from build123d import *

# Parameters (mm, degrees)
SKETCH1_R           = 10
SKETCH1_R_2         = 1
SKETCH1_R_3         = 1.5
BOSS_EXTRUDE1_DEPTH = 2
SKETCH2_R           = 4.5
SKETCH2_R_2         = 3.025
BOSS_EXTRUDE2_DEPTH = 2.5


with BuildPart() as part:
    # Sketch1 → Boss-Extrude1 (new body)
    with BuildSketch(Plane.XY):
        Circle(SKETCH1_R)
        with Locations((7, 0)):
            Circle(SKETCH1_R_2, mode=Mode.SUBTRACT)
        with Locations((0, 7)):
            Circle(SKETCH1_R_2, mode=Mode.SUBTRACT)
        Circle(SKETCH1_R_3, mode=Mode.SUBTRACT)
        with Locations((0, -7)):
            Circle(SKETCH1_R_2, mode=Mode.SUBTRACT)
        with Locations((-7, 0)):
            Circle(SKETCH1_R_2, mode=Mode.SUBTRACT)
    extrude(amount=BOSS_EXTRUDE1_DEPTH)

    # Sketch2 → Boss-Extrude2 (add)
    with BuildSketch(Plane.XY.offset(2)):
        Circle(SKETCH2_R)
        Circle(SKETCH2_R_2, mode=Mode.SUBTRACT)
    extrude(amount=BOSS_EXTRUDE2_DEPTH)


solid = part.part
CAD build for the part. Positions are in the model's coordinates, mm. A direction names the side the tool comes from. Give positions to 0.01 mm unless a question says otherwise; leave off trailing zeros. Write each loop counter-clockwise with the first axis right and the second up, starting at its lowest first coordinate (ties: lowest second). Pieces come first, ordered by that corner, then holes. Notation, with made-up numbers: M 2,5 L 23,5 A21 ccw 23,14 Z; hole C -32.5,81.5 d3. An arc over 180 degrees is marked long. Put each result on its own line as item: value. Start each with the question number.
(1) Band-saw the part on C-C, the plane y = -7. Write the cut outline in (x, z), and give its area (3 significant figures).
(2) Which spindle directions (+Z, -Z, +X, -X, +Y, -Y) get a long thin tool onto all of the face, cutting with end or side? Do faces 4 (the face through (2.794, -1.159, 3.232)), 5 (the face through (6.2, -0.6, 1)). Say none if no direction does.
(3) Probe L1, parallel to Y at x = 0, z = 0.7; L2, parallel to Y at x = 0, z = 3.8 (3 decimals); L3, parallel to Z at x = -4.75, y = 8. List the from-to ranges inside material, lowest first.
(4) Band-saw the part on A-A, the plane y = 0. Write the cut outline in (x, z) (3 decimals), and give its area (3 significant figures).
(5) Band-saw the part on D-D, the plane z = 0.4. Write the cut outline in (x, y), and give its area (3 significant figures).
(6) Flat gauge pins, fed straight in: pin 1 Ø1.5 at (x, z) = (3.5, 2.5) entering from -Y; pin 2 Ø1.5 at (x, y) = (-4.5, 7.5) entering from +Z; pin 3 Ø2 at (x, z) = (2, 2.5) entering from -Y. Where does each tip first touch, or does it go through?
(7) Mould opens along X. For faces 1 (the face through (0, -2, 0)), 2 (the face through (-1.5, 0.07, 0.99)), 3 (the face through (-0.59, 4.46, 3.23)) say: +X half, -X half, draft (parallel to the pull), parting line (faces both ways), or undercut.
Response values:
1. outline: M -7.14,0 L -1,0 L -1,2 L -7.14,2 Z; M 1,0 L 7.14,0 L 7.14,2 L 1,2 Z
1. area: 24.6 mm2
2. face 4: +Z
2. face 5: +Z, -Z
3. L1: y = -10 to -8, -6 to -1.5, 1.5 to 6, 8 to 10
3. L2: y = -4.5 to -3.025, 3.025 to 4.5
3. L3: z = 0 to 2
4. outline: M -10,0 L -8,0 L -8,2 L -10,2 Z; M -6,0 L -1.5,0 L -1.5,2 L -3.025,2 L -3.025,4.5 L -4.5,4.5 L -4.5,2 L -6,2 Z; M 1.5,0 L 6,0 L 6,2 L 4.5,2 L 4.5,4.5 L 3.025,4.5 L 3.025,2 L 1.5,2 Z; M 8,0 L 10,0 L 10,2 L 8,2 Z
4. area: 33.4 mm2
5. outline: C 0,0 d20; hole C -7,0 d2; hole C 0,0 d3; hole C 0,-7 d2; hole C 0,7 d2; hole C 7,0 d2
5. area: 295 mm2
6. pin 1: stops at y = -9.56
6. pin 2: stops at z = 2
6. pin 3: stops at y = -9.94
7. face 1: draft
7. face 2: undercut
7. face 3: parting line
